```python
from build123d import *

# Parameters (mm, degrees)
F0_W     = 1219.2
F0_H     = 914.4
F1_DEPTH = 304.8
F2_R     = 50.8
F3_DEPTH = 304.8


with BuildPart() as f1:
    # F0 (on Top) → F1 (new body)
    with BuildSketch(Plane.XY):
        Rectangle(F0_W, F0_H)
    extrude(amount=F1_DEPTH)

    # F2 (on face) → F3 (join)
    with BuildSketch(Plane.XY.offset(304.8)):
        with Locations((-457.2, 304.8)):
            Circle(F2_R)
        with Locations((457.2, 304.8)):
            Circle(F2_R)
        with Locations((457.2, -304.8)):
            Circle(F2_R)
        with Locations((-457.2, -304.8)):
            Circle(F2_R)
    extrude(amount=F3_DEPTH)


solid = f1.part
```
Could you check a few things on this model? Use its own coordinates, in mm. A direction names the side the tool comes from. Round coordinates to 2 decimals unless told otherwise and drop trailing zeros. Loops run counter-clockwise (first coordinate to the right, second up) from the corner with the lowest first, then second, coordinate; pieces in that order, holes last. Notation, with made-up numbers: (35, 67) -> (46, 67) arc R27 ccw to (46, 94) -> close; hole circle Ø4 at (25, -23). An arc over 180 degrees is marked (long way). One line per question, with ' | ' between items.
(1) For faces 4 (the face through (-9, 457.2, 150)), 5 (the face through (406.45, -302.57, 455.07)), which set-ups out of +Z, -Z, +X, -X, +Y, -Y let a thin tool reach every point of the face, with its end or its side?
Model answer:
face 4: +Z, -Z, +X, -X, +Y | face 5: +Z
(2) If we section it at B-B on x = 457.2: List the corners of the cut face in (y, z) for me, and give its area (3 significant figures).
Model answer:
outline: (-457.2, 0) -> (457.2, 0) -> (457.2, 304.8) -> (355.6, 304.8) -> (355.6, 609.6) -> (254, 609.6) -> (254, 304.8) -> (-254, 304.8) -> (-254, 609.6) -> (-355.6, 609.6) -> (-355.6, 304.8) -> (-457.2, 304.8) -> close | area: 341,000 mm^2
(3) If we section it at A-A on y = 304.8: List the corners of the cut face in (x, z) for me.
Model answer:
outline: (-609.6, 0) -> (609.6, 0) -> (609.6, 304.8) -> (508, 304.8) -> (508, 609.6) -> (406.4, 609.6) -> (406.4, 304.8) -> (-406.4, 304.8) -> (-406.4, 609.6) -> (-508, 609.6) -> (-508, 304.8) -> (-609.6, 304.8) -> close
(4) If we section it at D-D on x = 36.5: List the corners of the cut face in (y, z) for me.
Model answer:
outline: (-457.2, 0) -> (457.2, 0) -> (457.2, 304.8) -> (-457.2, 304.8) -> close
(5) Thinking about a two-plate mould opening in X: for faces 1 (the face through (416.887, 273.889, 455.066)), 2 (the face through (-609.6, -6, 150)), 3 (the face through (456, 306, 609.6)), which applies, released by +X, released by -X, zero draft, split by the parting line, or undercut?
Model answer:
face 1: undercut | face 2: released by -X | face 3: zero draft
(6) If we section it at C-C on z = 382: List the corners of the cut face in (x, y) for me.
Model answer:
outline: circle Ø101.6 at (-457.2, -304.8); circle Ø101.6 at (-457.2, 304.8); circle Ø101.6 at (457.2, -304.8); circle Ø101.6 at (457.2, 304.8)
(7) For pin 1 Ø8 at (x, y) = (376.5, 131.5) entering from +Z, with a flat end and sliding along its axis, tell me the tip position at first contact or that it passes through.
Model answer:
pin 1: stops at z = 304.8
(8) If I drill on probe 1 along Y at (x, z) = (-451.5, 565.5); probe 2 along Z at (x, y) = (278, 15); probe 3 along X at (y, z) = (-339, 557), over which ranges is the centre line in solid material (lowest first)?
Model answer:
probe 1: y = -355.28 to -254.32, 254.32 to 355.28 | probe 2: z = 0 to 304.8 | probe 3: x = -494.76 to -419.64, 419.64 to 494.76
